from build123d import *

# Parameters (mm, degrees)
SKETCH_1_W                = 40
SKETCH_1_H                = 10
EXTRUDE_1_DEPTH           = 8
HOLE_WIZARD_1_D           = 4.5
HOLE_WIZARD_1_CBORE_D     = 8
HOLE_WIZARD_1_CBORE_DEPTH = 4.6
HOLE_WIZARD_M4_1_D        = 3.3


with BuildPart() as part:
    # 草图1 → 凸台-拉伸1 (new body)
    with BuildSketch(Plane(origin=(0, 0, 0), x_dir=(1, 0, 0), z_dir=(0, 1, 0))):
        Rectangle(SKETCH_1_W, SKETCH_1_H)
    extrude(amount=EXTRUDE_1_DEPTH)

    # 打孔尺寸(%根据)内六角圆柱头螺钉的类型1 (through all)
    with Locations(Plane(origin=(0, 8, 0), x_dir=(1, 0, 0), z_dir=(0, 1, 0))):
        with Locations((14, 0), (-14, 0)):
            CounterBoreHole(HOLE_WIZARD_1_D / 2, HOLE_WIZARD_1_CBORE_D / 2, HOLE_WIZARD_1_CBORE_DEPTH)

    # M4 螺纹孔1 (through all)
    with Locations(Plane.XY.offset(5)):
        with Locations((0, 4)):
            Hole(HOLE_WIZARD_M4_1_D / 2)


solid = part.part
Geometry check sheet. Reference: the model listing, model coordinates, mm. A direction names the side the tool comes from. Round coordinates to 2 decimals unless told otherwise and drop trailing zeros. Order: outer loops, then holes, each group sorted by start corner. A loop starts at its lowest first (then second) coordinate and runs counter-clockwise, first axis right, second up. Notation, with made-up numbers: M 23,52.25 L 39,52.25 A21 cw 39,86.25 Z; hole C -8.5,0.5 d9. An arc over 180 degrees is marked long. Answer in a Markdown table with one row per item. Add a question column.
Item 1: Material ranges on L1, parallel to Y at x = 0, z = 0.25; L2, parallel to Z at x = 14, y = 5.1; L3, parallel to X at y = 1.75, z = 1, recorded low to high. Write a range as [from, to].
Item 2: Sectioned sample at C-C, the plane y = 4.75. Enter the section's corners in (x, z).
Item 3: Draft check along X on faces 3 (the face through (0, 2, -5)), 4 (the face through (20, 4, 0)), 5 (the face through (0.4, 2.4, -0.1)). Enter one of: released by +X, released by -X, zero draft, split by the parting line, or undercut.
Item 4: Depth check by flat-ended pin: pin 1 Ø5 at (x, z) = (14, 0) entering from +Y. Enter the tip coordinate at first touch or a pass-through.
Item 5: Set-up check for faces 1 (the face through (0, 2, 5)), 2 (the face through (10, 6, 0)): record each of +Z, -Z, +X, -X, +Y, -Y from which the full face is reachable in a straight line by a thin tool's end or side.
Item 6: Sectioned sample at A-A, the plane x = 0. Enter the section's corners in (y, z).
Item 7: Sectioned sample at B-B, the plane z = 1.25. Enter the section's corners in (x, y), plus the area to 3 significant figures.
Item 8: Sectioned sample at D-D, the plane x = 14. Enter the section's corners in (y, z).
Filled in:
| question | item | result |
|---|---|---|
| 1 | L1 | y = [0, 2.35], [5.65, 8] |
| 1 | L2 | z = [-5, -4], [4, 5] |
| 1 | L3 | x = [-20, -16.02], [-11.98, 11.98], [16.02, 20] |
| 2 | outline | M -20,-5 L -1.47,-5 L -1.47,5 L -20,5 Z; M 1.47,-5 L 20,-5 L 20,5 L 1.47,5 Z; hole C -14,0 d8; hole C 14,0 d8 |
| 3 | face 3 | zero draft |
| 3 | face 4 | released by +X |
| 3 | face 5 | undercut |
| 4 | pin 1 | stops at y = 3.4 |
| 5 | face 1 | +Z, +X, -X, +Y, -Y |
| 5 | face 2 | +Y |
| 6 | outline | M 0,-5 L 2.35,-5 L 2.35,5 L 0,5 Z; M 5.65,-5 L 8,-5 L 8,5 L 5.65,5 Z |
| 7 | outline | M -20,0 L -15.87,0 L -15.87,3.4 L -17.8,3.4 L -17.8,8 L -20,8 Z; M -12.13,0 L 12.13,0 L 12.13,3.4 L 10.2,3.4 L 10.2,8 L -10.2,8 L -10.2,3.4 L -12.13,3.4 Z; M 15.87,0 L 20,0 L 20,8 L 17.8,8 L 17.8,3.4 L 15.87,3.4 Z; hole C 0,4 d3.3 |
| 7 | area | 216 mm² |
| 8 | outline | M 0,-5 L 8,-5 L 8,-4 L 3.4,-4 L 3.4,-2.25 L 0,-2.25 Z; M 0,2.25 L 3.4,2.25 L 3.4,4 L 8,4 L 8,5 L 0,5 Z |
